Source: three-view drawing plus pictorial views. Frame: mm from the lowest corner of the part. A direction names the side the tool comes from. Give positions to 0.01 mm unless a question says otherwise; leave off trailing zeros. Loops run counter-clockwise (first coordinate to the right, second up) from the corner with the lowest first, then second, coordinate; pieces in that order, holes last. Notation, with made-up numbers: (20.25, 52.25) - (38.25, 52.25) arc R29 ccw to (38.25, 87.25) - close; hole circle Ø5 at (75, 67). An arc over 180 degrees is marked (long way). Answer as a JSON object with one key per item and string values. Group by question number.
(1) Material intervals for L1, parallel to Z at x = 1.6, y = 37; L2, parallel to X at y = 34.5, z = 69.5; L3, parallel to Y at x = 12.5, z = 23, sorted ascending.
(2) Mould query, pull axis X, two halves, no side actions, for the marked faces 1, 2, 3 and 4. Classes: +X half, -X half, draft (parallel to the pull), parting line (faces both ways), or undercut.
(3) Section query D-D (z = 38). Return loops of the section in (x, y), plus the area to 3 significant figures.
(4) Access query for the marked faces 5 and 6. Directions: +Z, -Z, +X, -X, +Y, -Y. A direction counts if a zero-diameter tool reaches every point of the face in a straight line with its end or side. Return the directions, or none.
(5) Section query B-B (z = 79.75). Count the separate pieces of the cut face and the enclosed holes in it, plus the area to 3 significant figures.
(6) Section query A-A (y = 17). Return loops of the section in (x, z), plus the area to 3 significant figures.
(7) Pin query (flat end, axial travel): P1, Ø2, axis at x = 21.5, z = 34.5, coming from the +Y side. Return the tip coordinate at first contact, or that it passes through.
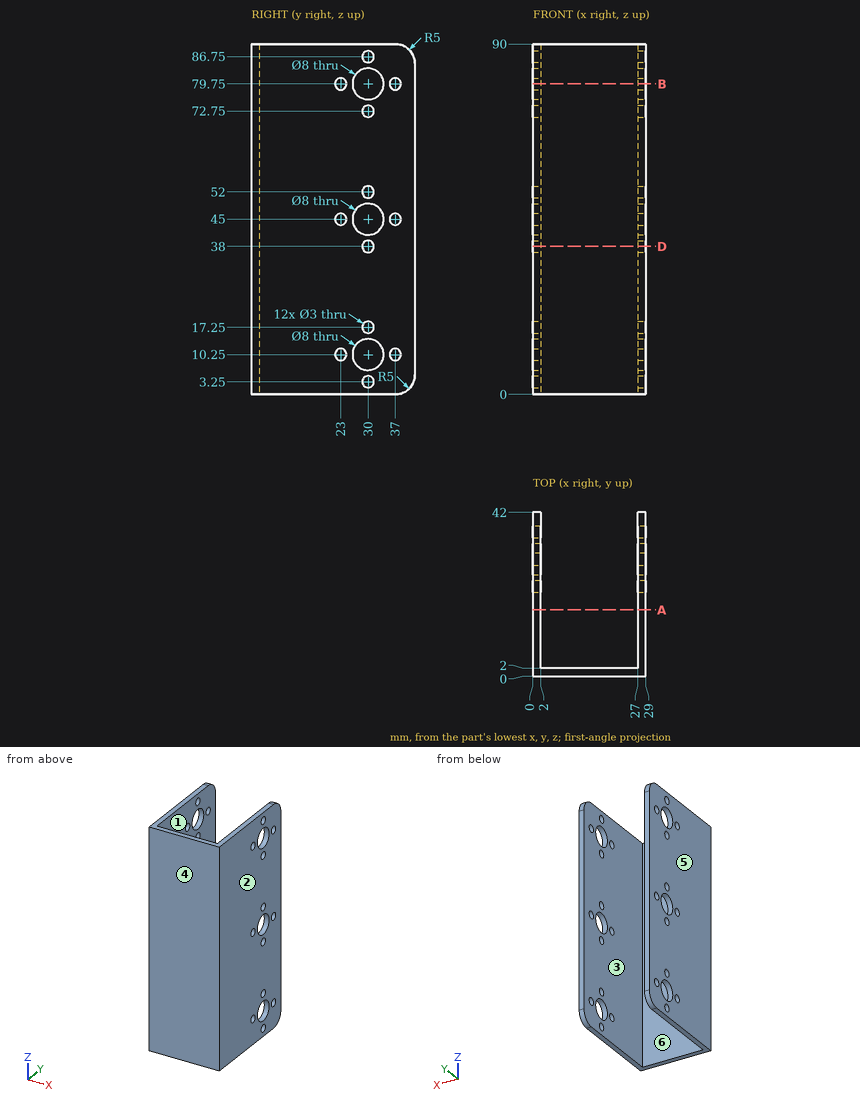
Recorded:
{
 "1": {"L1": "z = 0 to 8.75, 11.75 to 43.5, 46.5 to 78.25, 81.25 to 90", "L2": "x = 0 to 2, 27 to 29", "L3": "y = 0 to 2"},
 "2": {"face 1": "undercut", "face 2": "+X half", "face 3": "undercut", "face 4": "draft"},
 "3": {"outline": "(0, 0) - (29, 0) - (29, 28.5) - (27, 28.5) - (27, 2) - (2, 2) - (2, 28.5) - (0, 28.5) - close; (0, 31.5) - (2, 31.5) - (2, 42) - (0, 42) - close; (27, 31.5) - (29, 31.5) - (29, 42) - (27, 42) - close", "area": "206 mm^2"},
 "4": {"face 5": "+Z, -Z, -X, +Y, -Y", "face 6": "+Z, -Z, +Y"},
 "5": {"separate pieces": "7", "enclosed holes": "0", "area": "162 mm^2"},
 "6": {"outline": "(0, 0) - (2, 0) - (2, 90) - (0, 90) - close; (27, 0) - (29, 0) - (29, 90) - (27, 90) - close", "area": "360 mm^2"},
 "7": {"P1": "stops at y = 2"}
}
